Input: part model. Units: mm. Frame: model coordinates. Face numbers are marked on the shaded views. A direction names the side the tool comes from. Coordinates: 2 decimals unless noted, no trailing zeros. Order: outer loops, then holes, each group sorted by start corner. A loop starts at its lowest first (then second) coordinate and runs counter-clockwise, first axis right, second up.
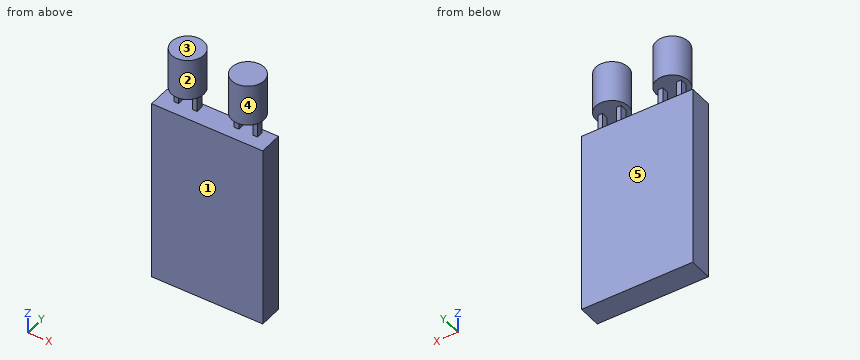
from build123d import *

# Parameters (mm, degrees)
SKETCH1_W           = 24
SKETCH1_H           = 40
BOSS_EXTRUDE1_DEPTH = 5
SKETCH2_W           = 1
SKETCH2_H           = 1.5
BOSS_EXTRUDE5_DEPTH = 44
SKETCH6_R           = 3.5
BOSS_EXTRUDE9_DEPTH = 9


with BuildPart() as part:
    # Sketch1 → Boss-Extrude1 (new body)
    with BuildSketch(Plane(origin=(0, 0, 0), x_dir=(1, 0, 0), z_dir=(0, 1, 0))):
        with Locations((-12, -10.571428571)):
            Rectangle(SKETCH1_W, SKETCH1_H)
    extrude(amount=BOSS_EXTRUDE1_DEPTH)

    # Sketch2 → Boss-Extrude5 (add)
    with BuildSketch(Plane(origin=(0, 0, -9.428571429), x_dir=(-1, 0, 0), z_dir=(0, 0, -1))):
        with Locations((3.5, 3.479518838)):
            Rectangle(SKETCH2_W, SKETCH2_H)
        with Locations((7.5, 3.479518838)):
            Rectangle(SKETCH2_W, SKETCH2_H)
        with Locations((16.5, 3.479518838)):
            Rectangle(SKETCH2_W, SKETCH2_H)
        with Locations((20.5, 3.479518838)):
            Rectangle(SKETCH2_W, SKETCH2_H)
    extrude(amount=-BOSS_EXTRUDE5_DEPTH)

    # Sketch6 → Boss-Extrude9 (add)
    with BuildSketch(Plane.XY.offset(34.571428571)):
        with Locations((-18.5, 3.40608753)):
            Circle(SKETCH6_R)
        with Locations((-5.5, 3.4)):
            Circle(SKETCH6_R)
    extrude(amount=BOSS_EXTRUDE9_DEPTH)


solid = part.part
Item 1: Cut plane B-B on x = -9.5. Return loops of the section in (y, z).
Response values:
outline: (0, -9.43) - (5, -9.43) - (5, 30.57) - (0, 30.57) - close
Item 2: Cut plane A-A on x = -18.5. Return loops of the section in (y, z), then the cut area to 3 significant figures.
Response values:
outline: (-0.09, 34.57) - (6.91, 34.57) - (6.91, 43.57) - (-0.09, 43.57) - close; (0, -9.43) - (5, -9.43) - (5, 30.57) - (0, 30.57) - close
area: 263 mm2
Item 3: Draft query along X for the marked faces 1 and 2. Return one class per face: pulls with the +X half, pulls with the -X half, needs draft (parallel to the pull), parting line crosses it, or undercut.
Response values:
face 1: needs draft
face 2: undercut
Item 4: Pin query (flat end, axial travel): pin 1 Ø1.5 at (x, z) = (-17.5, 5) entering from +Y; pin 2 Ø1.2 at (y, z) = (3.5, 32) entering from -X; pin 3 Ø4 at (x, y) = (-12, 6) entering from +Z. Return the tip coordinate at first contact, or that it passes through.
Response values:
pin 1: stops at y = 5
pin 2: stops at x = -21
pin 3: stops at z = 30.57
Item 5: Ray query, probe 1 along Z at (x, y) = (-8.25, 1.75); probe 2 along Y at (x, z) = (-21, 30); probe 3 along Z at (x, y) = (-13.5, 4). Return the intervals inside material, ascending.
Response values:
probe 1: z = -9.43 to 30.57, 34.57 to 43.57
probe 2: y = 0 to 5
probe 3: z = -9.43 to 30.57
Item 6: Cut plane C-C on z = -2. Return loops of the section in (x, y), then the cut area to 3 significant figures.
Response values:
outline: (-24, 0) - (0, 0) - (0, 5) - (-24, 5) - close
area: 120 mm2
Item 7: Access query for the marked faces 3, 4 and 5. Directions: +Z, -Z, +X, -X, +Y, -Y. A direction counts if a zero-diameter tool reaches every point of the face in a straight line with its end or side. Return the directions, or none.
Response values:
face 3: +Z, +X, -X, +Y, -Y
face 4: +Z
face 5: -Z, +X, -X, +Y
